Design review of the part built by this model. Coordinates are the model's own, in mm. A direction names the side the tool comes from. Coordinates: 2 decimals unless noted, no trailing zeros. Order: outer loops, then holes, each group sorted by start corner. A loop starts at its lowest first (then second) coordinate and runs counter-clockwise, first axis right, second up. Notation, with made-up numbers: (-11, -23.5) -> (12, -23.5) arc R18 ccw to (12, 5.5) -> close; hole circle Ø5 at (65.25, 20). An arc over 180 degrees is marked (long way). Write item = value, one per line.
Autodesk Fusion 360 part; units mm, degrees
sketch "Sketch1" plane through (0, 0, 0) normal (0, 1, 0) x (1, 0, 0)
  line L0 (0, 0) -> (45, 0) construction
  circle A0 centre (45, 0) radius 6.75
  circle A1 centre (0, 0) radius 6.75
  circle A2 centre (0, 0) radius 4.4
  circle A3 centre (45, 0) radius 4.4
  line L1 (-10, -10) -> (55, -10)
  line L2 (55, -10) -> (55, 10)
  line L3 (55, 10) -> (-10, 10)
  line L4 (-10, 10) -> (-10, -10)
  line L5 (22.5, -10) -> (22.5, 10) construction
  dimension "d1" = 45
  dimension "d2" = 8.8
  dimension "d3" = 13.5
  dimension "d4" = 20
  dimension "d5" = 65
sketch "Sketch2" plane through (0, 0, 0) normal (0, 0, 1) x (1, 0, 0)
  line L0 (55, 0) -> (-10, 0)
  line L1 (-10, 0) -> (-10, -60)
  line L2 (-10, -60) -> (55, -60)
  line L3 (55, -60) -> (55, 0)
  line L4 (15, -35) -> (55, -35)
  line L5 (15, -35) -> (15, -26.2815)
  line L6 (15, -26.2815) -> (25, -12)
  line L7 (25, -12) -> (25, 0)
  line L8 (0, 0) -> (45, 0)
  dimension "d6" = 60
  dimension "d7" = 10
  dimension "d8" = 25
  dimension "d9" = 25
  dimension "d10" = 145
  dimension "d11" = 12
extrude "Extrude1" add sketch "Sketch2" along normal up to surface (10 mm away) and the other way up to surface (10 mm away) contours L0 L1 L2 L3 L4 L5 L6 L7 L8
fillet "Fillet1" radius 5 12 edges at (25, -6, 10) (25, -6, -10) (-10, -30, -10) (-10, -30, 10) (55, -47.5, -10) (55, -47.5, 10) (20, -19.1407, 10) (20, -19.1407, -10) (25, -12, 0) (15, -30.6407, 10) (15, -30.6407, -10) (15, -26.2815, 0)
extrude "Extrude2" cut sketch "Sketch1" against normal through all contours A2 | A3
extrude "Extrude3" cut sketch "Sketch1" against normal blind 8 contours A1
extrude "Extrude4" cut sketch "Sketch1" against normal blind 8 from surface at -35 contours A0
chamfer "Chamfer1" distance 1 distance2 2 13 edges at (-10, 0, 0) (-8.5355, 0, -8.5355) (7.5, 0, -10) (23.5355, 0, -8.5355) (25, 0, 0) (23.5355, 0, 8.5355) (7.5, 0, 10) (-8.5355, 0, 8.5355) (30, -35, 10) (53.5355, -35, 8.5355) (55, -35, 0) (53.5355, -35, -8.5355) (30, -35, -10) measured on face at (-10, -20, -1.6667) measured on face at (-5.2379, -20, -9.9943) measured on face at (18.9167, 0, 0) measured on face at (24.9943, -6.949, -5.2379) measured on face at (25, -3.4745, -1.6667) measured on face at (24.9943, -6.949, 5.2379) measured on face at (18.9167, 0, 0) measured on face at (-9.9774, -40, 5.4753) measured on face at (22.75, -35, 0) measured on face at (50.2379, -51.6667, 9.9943) measured on face at (55, -51.6667, -1.6667) measured on face at (50.2379, -51.6667, -9.9943) measured on face at (22.75, -35, 0)
equation "d8 = 33 mm - 8 mm"
(1) For faces 1 (the flat face through (25, -6, 0)), 2 (the flat face through (30.3, -36, 9.5)), 3 (the cylindrical face through (14, -31, -8)), 4 (the cylindrical face through (-1.46, -3.94, 6.59)), 5 (the cylindrical face through (23, -6, 9)), list the 3-axis set-ups (+Z, -Z, +X, -X, +Y, -Y) from which the entire face can be reached by the end or side of a thin tool; tool diameter is ignored.
Report:
face_1 = +Z, -Z, +X, +Y
face_2 = +Z, +X
face_3 = -Z, +X
face_4 = +Y
face_5 = +Z, +X, +Y
(2) Insertion check: pin 1 (5.5 mm diameter, centred on x = 23.5, z = 2.5, fed in from +Y); pin 2 (2 mm diameter, centred on y = -29.5, z = -1.5, fed in from +X); pin 3 (4 mm diameter, centred on x = 41.5, z = -2.5, fed in from +Y); pin 4 (7 mm diameter, centred on x = -2, z = -2, fed in from +Y). Each pin has a flat end and moves straight along its axis. Give the tip position at first contact, or say it passes through.
Report:
pin_1 = 0
pin_2 = 15
pin_3 = -43
pin_4 = -8
(3) We need section A-A (x = 45). Write out the cut boundary in (y, z), and give its area (3 significant figures).
Report:
outline = (-60, -10) -> (-37, -10) -> (-35, -9) -> (-35, -6.75) -> (-43, -6.75) -> (-43, -4.4) -> (-60, -4.4) -> close; (-60, 4.4) -> (-43, 4.4) -> (-43, 6.75) -> (-35, 6.75) -> (-35, 9) -> (-37, 10) -> (-60, 10) -> close
area = 240 mm²
(4) For L1, parallel to X at y = -52.75, z = 0; L2, parallel to X at y = -3.5, z = 0; L3, parallel to X at y = -46.5, z = 0.75, list the stretches that pass through material, from the lowest coordinate up.
Report:
L1 = -10 to -4.4, 4.4 to 40.6, 49.4 to 55
L2 = -10 to -6.75, 6.75 to 25
L3 = -10 to -4.34, 4.34 to 40.66, 49.34 to 55
(5) We need section D-D (x = 0). Write out the cut boundary in (y, z).
Report:
outline = (-60, -10) -> (-1, -10) -> (0, -8) -> (0, -6.75) -> (-8, -6.75) -> (-8, -4.4) -> (-60, -4.4) -> close; (-60, 4.4) -> (-8, 4.4) -> (-8, 6.75) -> (0, 6.75) -> (0, 8) -> (-1, 10) -> (-60, 10) -> close
(6) The part is to be moulded in two halves that separate along X. For faces 6 (the flat face through (-9, -0.5, -0.1)), 7 (the cylindrical face through (18.83, -18.2, 8.57)), 8 (the cylindrical face through (4.197, -33.636, -1.322)), say which applies: released by +X, released by -X, zero draft, split by the parting line, or undercut.
Report:
face_6 = released by -X
face_7 = released by +X
face_8 = undercut
(7) We need section C-C (y = -45.5). Write out the cut boundary in (x, z).
Report:
outline = (-10, -5) arc R5 ccw to (-5, -10) -> (50, -10) arc R5 ccw to (55, -5) -> (55, 5) arc R5 ccw to (50, 10) -> (-5, 10) arc R5 ccw to (-10, 5) -> close; hole circle Ø8.8 at (0, 0); hole circle Ø8.8 at (45, 0)
(8) We need section B-B (z = 0). Give the number of separate pieces and of enclosed holes in the cut face, and give its area (3 significant figures).
Report:
separate_pieces = 3
enclosed_holes = 0
area = 1,870 mm²
